For this review, use the dimensioned drawing (mm, ordinates from the lowest corner) and the shaded views. Give positions to 0.01 mm unless a question says otherwise; leave off trailing zeros. Write each loop counter-clockwise with the first axis right and the second up, starting at its lowest first coordinate (ties: lowest second). Pieces come first, ordered by that corner, then holes.
1) We need section C-C on z = 1.35. Give the boundary of the cut face in (x, y), and give its area (3 significant figures).
2) We need section A-A on x = 5.7. Give the boundary of the cut face in (y, z).
3) Draft analysis for pull direction Y (two halves, no side actions). For the marked faces 1, 2 and 3, state which applies: pulls with the +Y half, pulls with the -Y half, needs draft (parallel to the pull), parting line crosses it, or undercut.
4) Wall thickness on line 1 along Y through (x, z) = (5.7, 1); line 2 along Y through (x, z) = (4.25, 1.8); line 3 along X through (y, z) = (7.25, 1.75): over which ranges is each line inside the solid? List them lowest first.
5) For P1, Ø4.5, axis at x = 5.7, y = 5.7, coming from the +Z side; P2, Ø1, axis at y = 7, z = 0.5, coming from the -X side, all flat-tipped, find the tip position at first contact; note any pin that passes through.
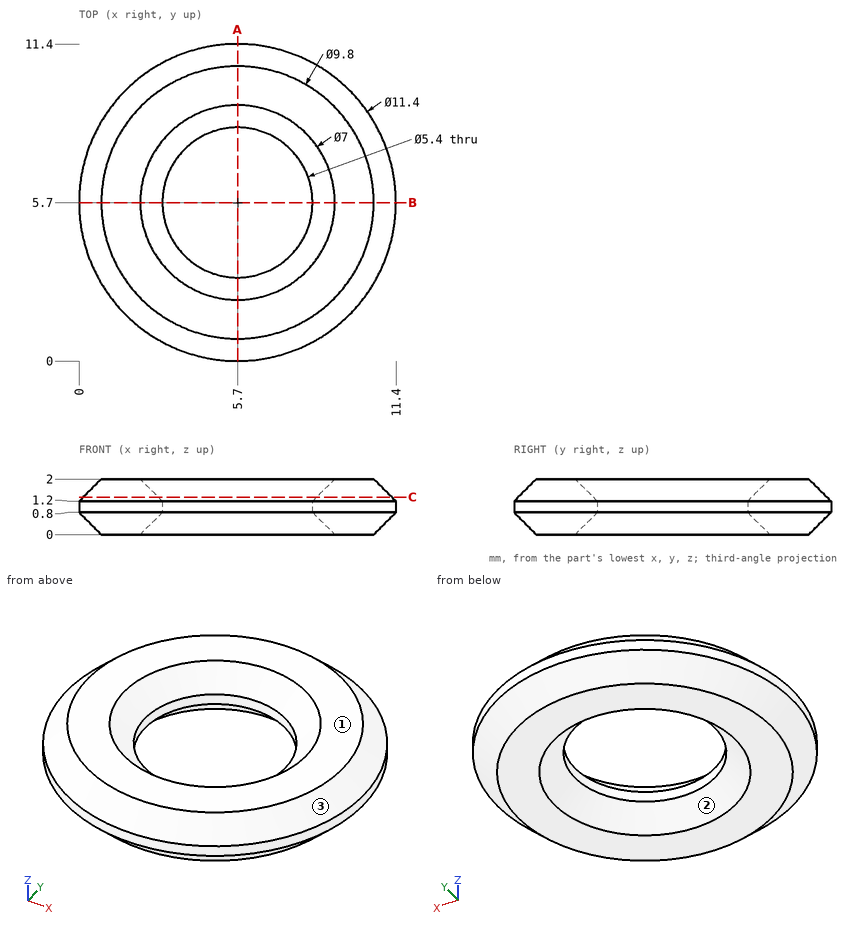
Results list:
1. outline: circle Ø11.1 at (5.7, 5.7); hole circle Ø5.7 at (5.7, 5.7)
1. area: 71.3 mm2
2. outline: (0, 0.8) - (0.8, 0) - (2.2, 0) - (3, 0.8) - (3, 1.2) - (2.2, 2) - (0.8, 2) - (0, 1.2) - close; (8.4, 0.8) - (9.2, 0) - (10.6, 0) - (11.4, 0.8) - (11.4, 1.2) - (10.6, 2) - (9.2, 2) - (8.4, 1.2) - close
3. face 1: needs draft
3. face 2: undercut
3. face 3: parting line crosses it
4. line 1: y = 0 to 3, 8.4 to 11.4
4. line 2: y = 0.81 to 2.74, 8.66 to 10.59
4. line 3: x = 0.79 to 2.84, 8.56 to 10.61
5. P1: passes through
5. P2: stops at x = 0.07
